Design review of the part built by this model. Coordinates are the model's own, in mm. A direction names the side the tool comes from. Round coordinates to 2 decimals unless told otherwise and drop trailing zeros. Order: outer loops, then holes, each group sorted by start corner. A loop starts at its lowest first (then second) coordinate and runs counter-clockwise, first axis right, second up.
from build123d import *

# Parameters (mm, degrees)
SKETCH1_R           = 2
SKETCH1_R_2         = 4.5
SKETCH1_R_3         = 3
BOSS_EXTRUDE2_DEPTH = 4
SKETCH1_8_R         = 4.5
CUT_EXTRUDE4_DEPTH  = 2


with BuildPart() as part:
    # Sketch1 → Boss-Extrude2 (new body)
    with BuildSketch(Plane(origin=(0, 0, 0), x_dir=(1, 0, 0), z_dir=(0, 1, 0))):
        with BuildLine():
            Line((21.446973136, 20), (-21.446973136, 20))
            ThreePointArc((-21.446973136, 20), (-23.935145745, 18.935145745), (-25, 16.446973136))
            Line((-25, 16.446973136), (-25, 16.276952121))
            Line((-25, 16.276952121), (-25, -16.276952121))
            Line((-25, -16.276952121), (-25, -16.446973136))
            ThreePointArc((-25, -16.446973136), (-23.935145745, -18.935145745), (-21.446973136, -20))
            Line((-21.446973136, -20), (21.446973136, -20))
            ThreePointArc((21.446973136, -20), (23.935145745, -18.935145745), (25, -16.446973136))
            Line((25, -16.446973136), (25, -16.276952121))
            Line((25, -16.276952121), (25, 16.276952121))
            Line((25, 16.276952121), (25, 16.446973136))
            ThreePointArc((25, 16.446973136), (23.935145745, 18.935145745), (21.446973136, 20))
        make_face()
        with Locations((-17.507214432, -2.825963154)):
            Circle(SKETCH1_R, mode=Mode.SUBTRACT)
        with Locations((17.492785568, -2.825963154)):
            Circle(SKETCH1_R, mode=Mode.SUBTRACT)
        with Locations((0, 5.276580282)):
            Circle(SKETCH1_R_2, mode=Mode.SUBTRACT)
        with Locations((0, 5.276580282)):
            Circle(SKETCH1_R_2)
        with Locations((0, 5.276580282)):
            Circle(SKETCH1_R_3, mode=Mode.SUBTRACT)
        with Locations((0, 5.276580282)):
            Circle(SKETCH1_R_3)
    extrude(amount=BOSS_EXTRUDE2_DEPTH)

    # Sketch1_8 → Cut-Extrude4 (cut)
    with BuildSketch(Plane(origin=(0, 0, 0), x_dir=(1, 0, 0), z_dir=(0, 1, 0))):
        with Locations((0, 5.276580282)):
            Circle(SKETCH1_8_R)
    extrude(amount=CUT_EXTRUDE4_DEPTH, mode=Mode.SUBTRACT)


solid = part.part
1) For faces 1 (the face through (0, 2, -5)), 2 (the face through (25, 2, 0)), list the 3-axis set-ups (+Z, -Z, +X, -X, +Y, -Y) from which the entire face can be reached by the end or side of a thin tool; tool diameter is ignored.
Results:
face 1: -Y
face 2: +Z, -Z, +X, +Y, -Y
2) Clearance check with flat-ended pins moving along their axes: P1, Ø2.5, axis at x = -17.51, z = 2.83, coming from the -Y side; P2, Ø3, axis at x = 18, z = 13.5, coming from the -Y side; P3, Ø4.5, axis at x = 2, z = -6, coming from the -Y side. State where each tip first meets the part, or that it passes through.
Results:
P1: passes through
P2: stops at y = 0
P3: stops at y = 2
3) The part is to be moulded in two halves that separate along X. For faces 3 (the face through (15.906, 1.972, 4.043)), 4 (the face through (-0.586, 0.986, -9.738)), 5 (the face through (0, 2, -20)), 6 (the face through (-23.91, 1.97, -18.96)), say which applies: released by +X, released by -X, zero draft, split by the parting line, or undercut.
Results:
face 3: undercut
face 4: undercut
face 5: zero draft
face 6: released by -X
4) Take a section at C-C on y = 3.1. Give the boundary of the cut face in (x, z).
Results:
outline: (-25, -16.45) arc R3.64 ccw to (-21.45, -20) - (21.45, -20) arc R3.64 ccw to (25, -16.45) - (25, 16.45) arc R3.64 ccw to (21.45, 20) - (-21.45, 20) arc R3.64 ccw to (-25, 16.45) - close; hole circle Ø4 at (-17.51, 2.83); hole circle Ø4 at (17.49, 2.83)
5) To check wall thickness, follow line 1 along X through (y, z) = (2.7, 3); line 2 along X through (y, z) = (0.85, -5); line 3 along Z through (x, y) = (0, 1.05). State the ranges of each line that lie inside material, in increasing order.
Results:
line 1: x = -25 to -19.5, -15.51 to 15.5, 19.49 to 25
line 2: x = -25 to -4.49, 4.49 to 25
line 3: z = -20 to -9.78, -0.78 to 20
6) Take a section at B-B on z = -8.5. Give the boundary of the cut face in (x, y), plus the area to 3 significant figures.
Results:
outline: (-25, 0) - (-3.14, 0) - (-3.14, 2) - (3.14, 2) - (3.14, 0) - (25, 0) - (25, 4) - (-25, 4) - close
area: 187 mm2
7) Take a section at A-A on x = 0. Give the boundary of the cut face in (y, z), plus the area to 3 significant figures.
Results:
outline: (0, -20) - (4, -20) - (4, 20) - (0, 20) - (0, -0.78) - (2, -0.78) - (2, -9.78) - (0, -9.78) - close
area: 142 mm2
